Can you work these out from the model? Positions are in its coordinate system, mm. A direction names the side the tool comes from. Coordinates: 2 decimals unless noted, no trailing zeros. Order: outer loops, then holes, each group sorted by start corner. A loop starts at its lowest first (then second) coordinate and runs counter-clockwise, first axis right, second up. Notation, with made-up numbers: (85.25, -8.75) - (103.25, -8.75) arc R7 cw to (103.25, 0.25) - close; hole circle Ø1 at (60, 40). An arc over 180 degrees is marked (long way). Return JSON: item names as keys, results as strings. Group by question number.
1) Imagine slicing it at B-B (x = 7). Write out the boundary of the cut face in (y, z) (3 decimals), and give its area (3 significant figures).
2) Imagine slicing it at A-A (z = -2.25). Write out the boundary of the cut face in (x, y), and give its area (3 significant figures).
3) Imagine slicing it at C-C (y = 5.5). Write out the boundary of the cut face in (x, z).
4) Which directions (+Z, -Z, +X, -X, +Y, -Y) give clear straight access to the entire face, cutting with the end or side of a thin tool? Please do faces 4 (the face through (1, 9, 3)), 5 (the face through (-0.867, 3.905, -2.958)).
5) Imagine slicing it at D-D (z = 1.5). Write out the boundary of the cut face in (x, y), and give its area (3 significant figures).
6) For pin 1 Ø2 at (x, y) = (0, 1.5) entering from +Z; pin 2 Ø1.5 at (x, z) = (6.5, -2.5) entering from -Y; pin 3 Ø1 at (x, y) = (7.5, -4) entering from -Z; pin 4 Ø5 at (x, z) = (2.5, -4) entering from +Y, each with a flat end and sliding along its axis, tell me the tip position at first contact or that it passes through.
7) If we mould it in two halves opening along Y, with no side actions, what happens to faces 1 (the face through (-0.08, 0.34, 0.49)), 2 (the face through (-2, 1, -6)), 3 (the face through (-2.17, -9.76, 1.48))? For each: pulls with the +Y half, pulls with the -Y half, needs draft (parallel to the pull), parting line crosses it, or undercut.
8) If I drill on line 1 along Y through (x, z) = (0, -4.15); line 2 along Z through (x, y) = (6.75, -6.25); line 3 along Y through (x, z) = (-2.25, 2.75), over which ranges is the centre line in solid material (lowest first)?
```python
from build123d import *

# Parameters (mm, degrees)
F0_R     = 10
F1_DEPTH = 3
F4_R     = 4
F5_DEPTH = 6
F7_D     = 4
F7_DEPTH = 5.5
F7_TIP   = 1.2017212381


with BuildPart() as f1:
    # F0 (on Top) → F1 (new body)
    with BuildSketch(Plane.XY):
        Circle(F0_R)
    extrude(amount=F1_DEPTH)

    # F2 (on Front) → F3 (revolve, cut)
    with BuildSketch(Plane.XZ):
        with BuildLine():
            Line((0, 1), (0, 41))
            ThreePointArc((0, 41), (-20, 21), (0, 1))
        make_face()
    revolve(axis=Axis((0, 0, 27.4340542965), (0, 0, -1)), mode=Mode.SUBTRACT)

    # F4 (on face) → F5 (join)
    with BuildSketch(Plane(origin=(0, 0, 0), x_dir=(1, 0, 0), z_dir=(0, 0, -1))):
        Circle(F4_R)
    extrude(amount=F5_DEPTH)

    # F7
    with Locations(Plane(origin=(0, 0, -6), x_dir=(1, 0, 0), z_dir=(0, 0, -1))):
        with Locations((0, 0)):
            Hole(F7_D / 2, depth=F7_DEPTH)
            with Locations((0, 0, -(F7_DEPTH + F7_TIP / 2))):  # 118° drill point
                Cone(0, F7_D / 2, F7_TIP, mode=Mode.SUBTRACT)


solid = f1.part
```
Calculated:
{
 "1": {"outline": "(-7.141, 0) - (7.141, 0) - (7.141, 3) - (5.196, 3) arc R18.735 cw to (-5.196, 3) - (-7.141, 3) - close", "area": "37.7 mm2"},
 "2": {"outline": "circle Ø8 at (0, 0); hole circle Ø4 at (0, 0)", "area": "37.7 mm2"},
 "3": {"outline": "(-8.35, 0) - (8.35, 0) - (8.35, 3) - (6.76, 3) arc R19.23 cw to (-6.76, 3) - (-8.35, 3) - close"},
 "4": {"face 4": "+Z, +X, -X, +Y, -Y", "face 5": "-Z"},
 "5": {"outline": "circle Ø20 at (0, 0); hole circle Ø8.89 at (0, 0)", "area": "252 mm2"},
 "6": {"pin 1": "z = 1.16", "pin 2": "through", "pin 3": "z = 0", "pin 4": "y = 4"},
 "7": {"face 1": "undercut", "face 2": "needs draft", "face 3": "parting line crosses it"},
 "8": {"line 1": "-4 to -2, 2 to 4", "line 2": "0 to 3", "line 3": "-9.74 to -7.87, 7.87 to 9.74"}
}
